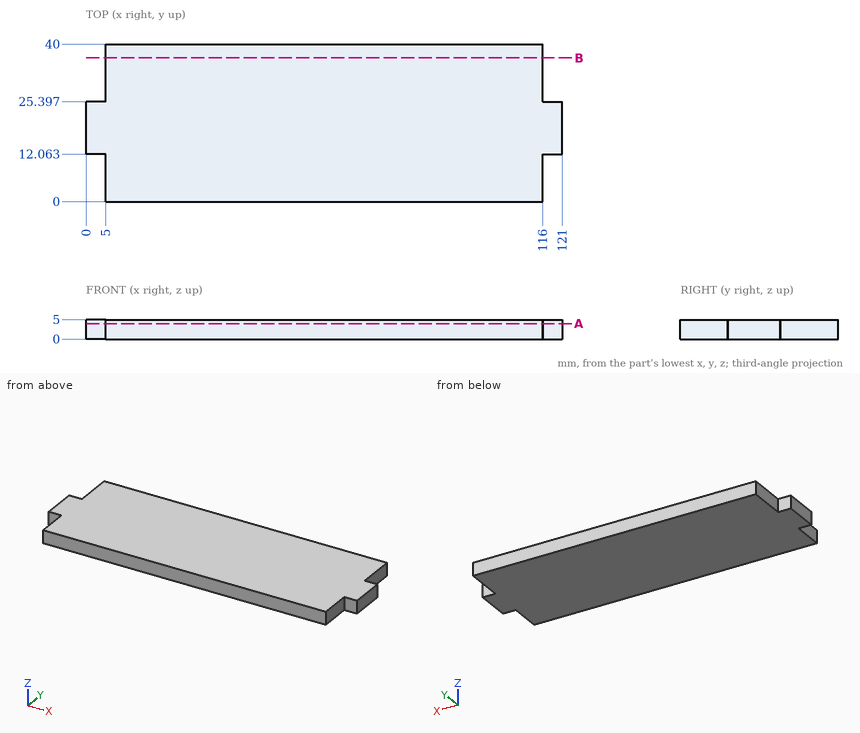
Check sheet for the drawn part. Datum: minimum x, y, z corner. Units: mm. Round coordinates to 2 decimals unless told otherwise and drop trailing zeros. Order: outer loops, then holes, each group sorted by start corner. A loop starts at its lowest first (then second) coordinate and runs counter-clockwise, first axis right, second up.
1) Section check A-A (z = 3.95). Record the boundary of the cut face in (x, y), and give its area (3 significant figures).
2) Scan line: line 1 (X direction, y = 37.5, z = 1.9). Record every from-to range of solid material in increasing order.
3) Section check B-B (y = 36.5). Record the boundary of the cut face in (x, z), and give its area (3 significant figures).
4) Go/stop test with flat-tipped pins: pin 1 Ø1.5 at (x, z) = (3, 2.5) entering from +Y; pin 2 Ø2.5 at (y, z) = (4, 3.5) entering from -X; pin 3 Ø1.5 at (y, z) = (4, 2) entering from +X. Record where each tip stops, or that it passes through.
Result:
1. outline: (0, 12.06) - (5, 12.06) - (5, 0) - (116, 0) - (116, 12.06) - (121, 12.06) - (121, 25.4) - (116, 25.4) - (116, 40) - (5, 40) - (5, 25.4) - (0, 25.4) - close
1. area: 4,570 mm2
2. line 1: x = 5 to 116
3. outline: (5, 0) - (116, 0) - (116, 5) - (5, 5) - close
3. area: 555 mm2
4. pin 1: stops at y = 25.4
4. pin 2: stops at x = 5
4. pin 3: stops at x = 116
